Part model, mm, in its own coordinate system. A direction names the side the tool comes from. Coordinates: 2 decimals unless noted, no trailing zeros. Loops run counter-clockwise (first coordinate to the right, second up) from the corner with the lowest first, then second, coordinate; pieces in that order, holes last. Notation, with made-up numbers: (62.5, 71) -> (67.5, 71) arc R27 ccw to (67.5, 109) -> close; hole circle Ø9 at (-33, 61). An arc over 180 degrees is marked (long way). One line per question, with ' | ' between items. Start each with the question number.
1) Cut at A-A (z = 0). List the corners of the cut face in (x, y), plus the area to 3 significant figures.
2) Probe L1, parallel to Y at x = 35, z = -0.05; L2, parallel to Z at x = 8, y = -1.85; L3, parallel to X at y = -0.5, z = 0.45. List the from-to ranges inside material, lowest first. Write a range as from..to.
3) 3-axis set-ups, long thin cutter, end or side, ignore diameter. For faces 4 (the face through (0.51, -0.49, 0.63)), 5 (the face through (32, -2.58, 0.17)), 6 (the face through (63.25, 0, 0)): which of +Z, -Z, +X, -X, +Y, -Y reach the whole face in a straight line?
4) Two-plate mould, pull along X, no slides. Class faces 1 (the face through (62.76, -0.49, 0.63)), 2 (the face through (0, 0, 0)), 3 (the face through (59.84, -0.22, 0.1)): released by +X, released by -X, zero draft, split by the parting line, or undercut.
5) Cut at B-B (x = 55.5). List the corners of the cut face in (y, z), plus the area to 3 significant figures.
from build123d import *

# Parameters (mm, degrees)
SKETCH1_R = 0.8


with BuildPart() as part:
    # Sweep1: sweep along a path in Sketch2
    with BuildLine(Plane.XY) as sweep1_path:
        Line((0, 0), (1, 0))
        ThreePointArc((1, 0), (1.55762039, -0.079307546), (2.071017274, -0.310940499))
        Line((2.071017274, -0.310940499), (3.928982726, -1.489059501))
        ThreePointArc((3.928982726, -1.489059501), (4.44237961, -1.720692454), (5, -1.8))
        Line((5, -1.8), (58.25, -1.8))
        ThreePointArc((58.25, -1.8), (58.80762039, -1.720692454), (59.321017274, -1.489059501))
        Line((59.321017274, -1.489059501), (61.178982726, -0.310940499))
        ThreePointArc((61.178982726, -0.310940499), (61.69237961, -0.079307546), (62.25, 0))
        Line((62.25, 0), (63.25, 0))
    # Sketch1 → Sweep1 (sweep)
    with BuildSketch(Plane(origin=(0, 0, 0), x_dir=(0, 0, -1), z_dir=(1, 0, 0))):
        Circle(SKETCH1_R)
    sweep(path=sweep1_path.line)


solid = part.part
Reported:
1) outline: (0, -0.8) -> (1, -0.8) arc R1.2 cw to (1.64, -0.99) -> (3.5, -2.16) arc R2.8 ccw to (5, -2.6) -> (58.25, -2.6) arc R2.8 ccw to (59.75, -2.16) -> (61.61, -0.99) arc R1.2 cw to (62.25, -0.8) -> (63.25, -0.8) -> (63.25, 0.8) -> (62.25, 0.8) arc R2.8 ccw to (60.75, 0.36) -> (58.89, -0.81) arc R1.2 cw to (58.25, -1) -> (5, -1) arc R1.2 cw to (4.36, -0.81) -> (2.5, 0.36) arc R2.8 ccw to (1, 0.8) -> (0, 0.8) -> close | area: 103 mm²
2) L1: y = -2.6..-1 | L2: z = -0.8..0.8 | L3: x = 0..3.6, 59.65..63.25
3) face 4: -X | face 5: none | face 6: +Z, -Z, +X, +Y, -Y
4) face 1: zero draft | face 2: released by -X | face 3: undercut
5) outline: circle Ø1.6 at (-1.8, 0) | area: 2.01 mm²
